The listing builds one solid part. Answer for the finished solid, in the listing's coordinates (mm). Face numbers are marked on the shaded views. Give positions to 0.01 mm unless a question says otherwise; leave off trailing zeros. Write each loop counter-clockwise with the first axis right and the second up, starting at its lowest first coordinate (ties: lowest second). Pieces come first, ordered by that corner, then holes. Notation, with made-up numbers: (26, 31.5) - (42, 31.5) arc R19 ccw to (42, 62.5) - close; hole circle Ø10 at (-12.75, 25.5). An arc over 180 degrees is marked (long way). One line per question, with ' | ' between items. Start each with the question number.
1. The mould has two halves that part along Z. Classify the marked faces 1, 2 and 3: +Z half, -Z half, draft (parallel to the pull), parting line (faces both ways), or undercut.
2. A cutting plane is placed at A-A (z = 0). Determine the outline of the cut face in (x, y) (3 decimals), then the cut area to 3 significant figures.
3. Find the intervals of material crossed by L1, parallel to X at y = 1.5, z = -0.05; L2, parallel to Z at x = 0.15, y = 6.75; L3, parallel to Z at x = -1.15, y = 2.5, in increasing order. Write a range as from..to.
4. A cutting plane is placed at B-B (y = 0.5). Determine the outline of the cut face in (x, z) (3 decimals), then the cut area to 3 significant figures.
5. A cutting plane is placed at C-C (x = -0.5). Determine the outline of the cut face in (y, z).
6. Given P1, Ø2, axis at x = -2, z = 2, coming from the +Y side; P2, Ø1.5, axis at x = -2, y = 8.5, coming from the +Z side, each flat-ended and moving along its own axis, determine where each tip first touches the part or whether it passes through.
7. A cutting plane is placed at D-D (z = -1.7). Determine the outline of the cut face in (x, y), then the cut area to 3 significant figures.
Autodesk Inventor part; units mm, degrees
ref_plane "YZ Plane" through (0, 0, 0) normal (1, 0, 0) x (0, 1, 0)
ref_plane "XZ Plane" through (0, 0, 0) normal (0, 1, 0) x (-1, 0, 0)
ref_plane "XY Plane" through (0, 0, 0) normal (0, 0, 1) x (1, 0, 0)
sketch "Boceto1" plane through (0, 0, 0) normal (0, 1, 0) x (-1, 0, 0)
  circle A0 centre (0, 0) radius 1.375
  circle A1 centre (0, 0) radius 3
  line L0 (0, -3) -> (-2.5981, -1.5)
  line L1 (-2.5981, -1.5) -> (-2.5981, 1.5)
  line L2 (-2.5981, 1.5) -> (0, 3)
  line L3 (0, 3) -> (2.5981, 1.5)
  line L4 (2.5981, 1.5) -> (2.5981, -1.5)
  line L5 (2.5981, -1.5) -> (0, -3)
  dimension "d1" = 6
  dimension "d0" = 2.75
extrude "Extrusión1" add sketch "Boceto1" along normal blind 9.5 contours L4 L5 L0 L1 L2 L3
properties part number "Espaciador"
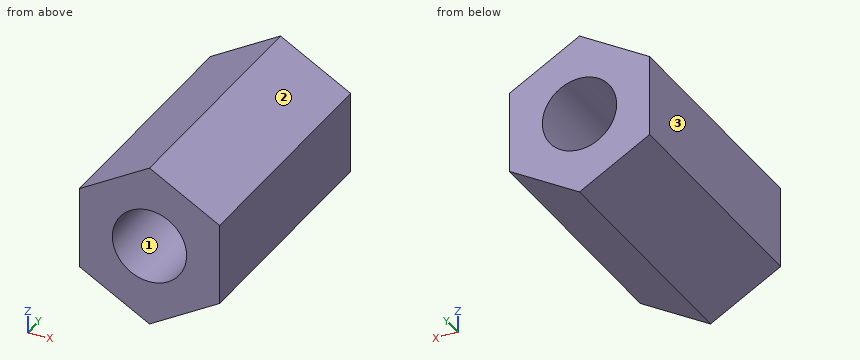
Determined:
1) face 1: undercut | face 2: +Z half | face 3: draft
2) outline: (-2.598, 0) - (-1.375, 0) - (-1.375, 9.5) - (-2.598, 9.5) - close; (1.375, 0) - (2.598, 0) - (2.598, 9.5) - (1.375, 9.5) - close | area: 23.2 mm2
3) L1: -2.6..-1.37, 1.37..2.6 | L2: -2.91..-1.37, 1.37..2.91 | L3: -2.34..-0.75, 0.75..2.34
4) outline: (-2.598, -1.5) - (0, -3) - (2.598, -1.5) - (2.598, 1.5) - (0, 3) - (-2.598, 1.5) - close; hole circle Ø2.75 at (0, 0) | area: 17.4 mm2
5) outline: (0, -2.71) - (9.5, -2.71) - (9.5, -1.28) - (0, -1.28) - close; (0, 1.28) - (9.5, 1.28) - (9.5, 2.71) - (0, 2.71) - close
6) P1: y = 9.5 | P2: z = 2.28
7) outline: (-2.25, 0) - (2.25, 0) - (2.25, 9.5) - (-2.25, 9.5) - close | area: 42.8 mm2
